The listing builds one solid part. Answer for the finished solid, in the listing's coordinates (mm). A direction names the side the tool comes from. Give positions to 0.01 mm unless a question says otherwise; leave off trailing zeros. Write each loop counter-clockwise with the first axis right and the second up, starting at its lowest first coordinate (ties: lowest second). Pieces come first, ordered by that corner, then holes. Notation, with made-up numbers: M 38.25,89 L 46.25,89 A14 cw 46.25,94 Z; hole C -25,-38.75 d11. An arc over 180 degrees is marked long. Answer as a JSON object with one key per item and string values.
```python
from build123d import *

# Parameters (mm, degrees)
EXTRUDE_THIN1_START = -11.1125
EXTRUDE_THIN1_DEPTH = 22.225
EXTRUDE4_START      = -3.556
EXTRUDE4_DEPTH      = 3.556
SKETCH4_R           = 2.0828
CUT_EXTRUDE1_DEPTH  = 34.3375
CUT_EXTRUDE2_DEPTH  = 32.080055377
CHAMFER1_SIZE       = 2.286


# Read off the part's stored shape, not the designer's step: Extrude-Thin1
with BuildPart() as part:
    # Extrude-Thin1 outline → Extrude-Thin1 (new body)
    with BuildSketch(Plane(origin=(0, 0, 0), x_dir=(1, 0, 0), z_dir=(0, 1, 0)).offset(EXTRUDE_THIN1_START)):
        with BuildLine():
            Line((3.9116, -3.556), (22.225, -3.556))
            Line((22.225, -3.556), (22.225, 0))
            Line((22.225, 0), (3.9116, 0))
            ThreePointArc((3.9116, 0), (1.145681115, -1.145681115), (0, -3.9116))
            Line((0, -3.9116), (0, -22.225))
            Line((0, -22.225), (3.556, -22.225))
            Line((3.556, -22.225), (3.556, -3.9116))
            ThreePointArc((3.556, -3.9116), (3.660152829, -3.660152829), (3.9116, -3.556))
        make_face()
    extrude(amount=EXTRUDE_THIN1_DEPTH)

    # Sketch5 → Extrude4 (add)
    with BuildSketch(Plane(origin=(0, 11.1125, 0), x_dir=(1, 0, 0), z_dir=(0, 1, 0)).offset(EXTRUDE4_START)):
        with BuildLine():
            Line((3.9116, -3.556), (19.685, -3.556))
            ThreePointArc((19.685, -3.556), (8.902403387, -8.902403387), (3.556, -19.685))
            Line((3.556, -19.685), (3.556, -3.9116))
            ThreePointArc((3.556, -3.9116), (3.660152829, -3.660152829), (3.9116, -3.556))
        make_face()
    extrude4 = extrude(amount=EXTRUDE4_DEPTH)

    # Mirror2: Extrude4 across plane
    add(extrude4.mirror(Plane.ZX))

    # Sketch4 → Cut-Extrude1 (cut, through all)
    with BuildSketch(Plane(origin=(0, 0, 0), x_dir=(0, 0, -1), z_dir=(1, 0, 0))):
        with Locations(Location((-16.225, 0, 0), (0, 0, 180))):
            Circle(SKETCH4_R)
    cut_extrude1 = extrude(amount=CUT_EXTRUDE1_DEPTH, mode=Mode.SUBTRACT)

    # Sketch6 → Cut-Extrude2 (cut, symmetric)
    with BuildSketch(Plane(origin=(3.556, 0, 0), x_dir=(0, 0, -1), z_dir=(1, 0, 0))):
        with BuildLine():
            Line((10.456138589, 73.60153911), (-19.685, 11.1125))
            ThreePointArc((-19.685, 11.1125), (-22.225, 0), (-19.685, -11.1125))
            Line((-19.685, -11.1125), (10.456138589, -73.60153911))
            Line((10.456138589, -73.60153911), (-128.300745843, -73.60153911))
            Line((-128.300745843, -73.60153911), (-128.300745843, 73.60153911))
            Line((-128.300745843, 73.60153911), (10.456138589, 73.60153911))
        make_face()
    cut_extrude2 = extrude(amount=CUT_EXTRUDE2_DEPTH, both=True, mode=Mode.SUBTRACT)

    # Mirror3: Cut-Extrude1, Cut-Extrude2 across plane
    add(cut_extrude1.mirror(Plane(origin=(0, 0, 0), x_dir=(0.7071067811865465, 0, 0.7071067811865486), z_dir=(-0.7071067811865488, 0, 0.7071067811865464))), mode=Mode.SUBTRACT)
    add(cut_extrude2.mirror(Plane(origin=(0, 0, 0), x_dir=(0.7071067811865465, 0, 0.7071067811865486), z_dir=(-0.7071067811865488, 0, 0.7071067811865464))), mode=Mode.SUBTRACT)

    # Chamfer1
    chamfer1_edges = [part.edges().sort_by_distance(p)[0] for p in [
        (3.556, 0, 14.1422),
        (14.1422, 0, 3.556),
    ]]
    chamfer(chamfer1_edges, length=CHAMFER1_SIZE)


solid = part.part
```
1. For faces 5 (the flat face through (7, 7.557, 8)), 6 (the cylindrical face through (9.024, -9.31, 8.782)), determine the directions among +Z, -Z, +X, -X, +Y, -Y from which every point of the face is accessible in a straight line to the end or side of a thin tool.
Verdict:
{"face 5": "+Z, +X", "face 6": "+Z, +X, +Y, -Y"}
2. A cutting plane is placed at A-A, the plane y = 0. Give the vertices of the cut face in (x, z) (3 decimals).
Verdict:
{"outline": "M 0,3.912 A3.912 ccw 3.912,0 L 14.142,0 L 14.142,1.27 L 11.856,3.556 L 3.912,3.556 A0.356 cw 3.556,3.912 L 3.556,11.856 L 1.27,14.142 L 0,14.142 Z; M 0,18.308 L 1.27,18.308 L 3.556,20.594 L 3.556,22.225 L 0,22.225 Z; M 18.308,0 L 22.225,0 L 22.225,3.556 L 20.594,3.556 L 18.308,1.27 Z"}
3. Flat-ended cylindrical pins translate along their axes: pin 1 (1 mm diameter, centred on y = -7.5, z = 9.5, fed in from +X); pin 2 (3.5 mm diameter, centred on x = 16.225, y = 0, fed in from -Z); pin 3 (1 mm diameter, centred on x = 9, y = 7.5, fed in from +Z); pin 4 (5 mm diameter, centred on x = 11, y = 0, fed in from +Z). Find the tip coordinate at first contact, or state that the pin passes through.
Verdict:
{"pin 1": "stops at x = 8.8", "pin 2": "passes through", "pin 3": "stops at z = 9.31", "pin 4": "stops at z = 3.56"}
4. Consider line 1 along Y through (x, z) = (9.5, 4); line 2 along X through (y, z) = (-7.75, 20). Determine where each line is inside the solid, lowest interval first.
Verdict:
{"line 1": "y = -11.11 to -7.56, 7.56 to 11.11", "line 2": "x = 0 to 3.56"}
5. A cutting plane is placed at B-B, the plane z = 9.75. Give the vertices of the cut face in (x, y).
Verdict:
{"outline": "M 0,-11.11 L 8.11,-11.11 L 8.11,-7.56 L 3.56,-7.56 L 3.56,7.56 L 8.11,7.56 L 8.11,11.11 L 0,11.11 Z"}
6. The mould has two halves that part along X. Classify faces 1 (the flat face through (13, 0, 0)), 2 (the cylindrical face through (14.144, -0.092, 0.626)), 3 (the conical face through (14.001, -0.098, 1.413)), 4 (the flat face through (0, 0, 13)): released by +X, released by -X, zero draft, split by the parting line, or undercut.
Verdict:
{"face 1": "zero draft", "face 2": "undercut", "face 3": "undercut", "face 4": "released by -X"}
7. A cutting plane is placed at C-C, the plane x = 11.25. Give the vertices of the cut face in (y, z).
Verdict:
{"outline": "M -11.11,0 L 11.11,0 L 11.11,6.91 L 7.56,6.91 L 7.56,3.56 L -7.56,3.56 L -7.56,6.91 L -11.11,6.91 Z"}
